The figure shows three views and two pictorial views of one solid part (mm, origin at its lowest corner). Answer the questions. Round coordinates to 2 decimals unless told otherwise and drop trailing zeros. Order: outer loops, then holes, each group sorted by start corner. A loop starts at its lowest first (then second) coordinate and runs counter-clockwise, first axis right, second up. Notation, with made-up numbers: (-39, -32.5) - (-1, -32.5) arc R17 cw to (-1, -19.5) - close; hole circle Ø6 at (48.5, -8.5). An arc over 180 degrees is marked (long way). Write item = value, one per line.
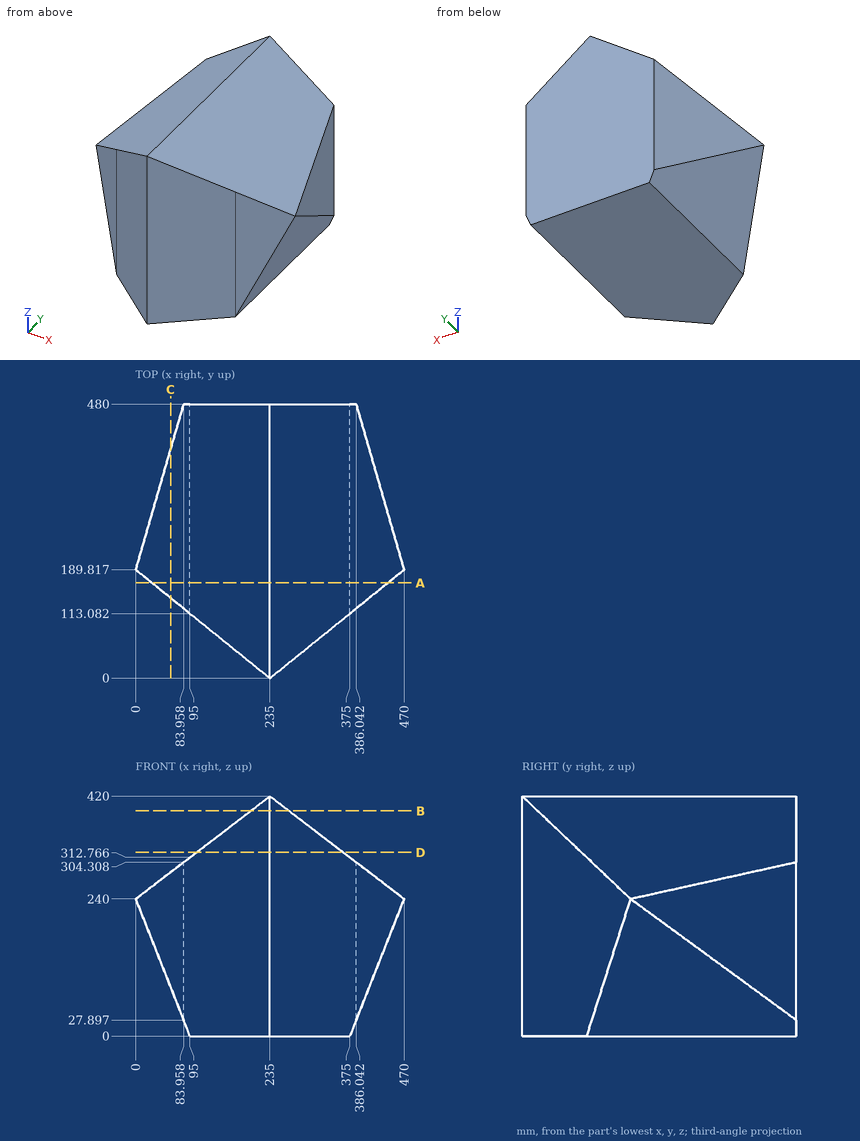
Q1. Section C-C on x = 61 is taken. Determine the outline of the cut face in (y, z) (1 decimal), then the cut area to 3 significant figures.
Model answer:
outline = (140.5, 85.9) - (400.7, 85.9) - (400.7, 286.7) - (140.5, 286.7) - close
area = 52,200 mm^2
Q2. Section B-B on z = 394 is taken. Determine the outline of the cut face in (x, y) (1 decimal), then the cut area to 3 significant figures.
Model answer:
outline = (201.1, 27.4) - (235, 0) - (268.9, 27.4) - (268.9, 480) - (201.1, 480) - close
area = 31,700 mm^2
Q3. Flat-ended cylindrical pins translate along their axes: P1, Ø2, axis at y = 418, z = 319, coming from the +X side (1 decimal); P2, Ø10, axis at y = 295.5, z = 220, coming from the +X side; P3, Ø12, axis at x = 338.5, z = 139, coming from the -Y side (1 decimal); P4, Ø1, axis at x = 116.5, y = 155, coming from the -Z side. Find the tip coordinate at first contact, or state that the pin passes through.
Model answer:
P1 = 368.2
P2 = 440.87
P3 = 78.8
P4 = 0
Q4. Section D-D on z = 321.5 is taken. Determine the outline of the cut face in (x, y).
Model answer:
outline = (106.4, 103.87) - (235, 0) - (363.6, 103.87) - (363.6, 480) - (106.4, 480) - close
Q5. Find the intervals of material crossed by line 1 (Y direction, x = 125.5, z = 22) (1 decimal); line 2 (Z direction, x = 176.5, y = 360); line 3 (X direction, y = 313.5, z = 116.5) (1 decimal), in increasing order. Write a range as from..to.
Model answer:
line_1 = 88.4..480
line_2 = 0..375.19
line_3 = 48.9..421.1
Q6. Section A-A on y = 167 is taken. Determine the outline of the cut face in (x, z).
Model answer:
outline = (28.25, 168.64) - (95, 0) - (375, 0) - (441.75, 168.64) - (441.75, 261.64) - (235, 420) - (28.25, 261.64) - close
